from build123d import *

# Parameters (mm, degrees)
F0_W     = 148
F0_H     = 118
F1_DEPTH = 59
F2_R     = 25.75
F3_DEPTH = 50
F2_R_2   = 18
F4_DEPTH = 40
F2_R_3   = 12.5
F5_DEPTH = 38.5
F2_R_4   = 5.4
F6_DEPTH = 38.3


with BuildPart() as f1:
    # F0 (on Top) → F1 (new body)
    with BuildSketch(Plane.XY):
        Rectangle(F0_W, F0_H)
    extrude(amount=F1_DEPTH)

    # F2 (on face) → F3 (cut)
    with BuildSketch(Plane.XY.offset(59)):
        with Locations((0, -26)):
            Circle(F2_R)
    extrude(amount=-F3_DEPTH, mode=Mode.SUBTRACT)

    # F2 (on face) → F4 (cut)
    with BuildSketch(Plane.XY.offset(59)):
        with Locations((-51, 36)):
            Circle(F2_R_2)
        with Locations((0, 36)):
            Circle(F2_R_2)
        with Locations((51, 36)):
            Circle(F2_R_2)
    extrude(amount=-F4_DEPTH, mode=Mode.SUBTRACT)

    # F2 (on face) → F5 (cut)
    with BuildSketch(Plane.XY.offset(59)):
        with Locations((-51, 0)):
            Circle(F2_R_3)
        with Locations((-51, -36)):
            Circle(F2_R_3)
        with Locations((51, 0)):
            Circle(F2_R_3)
        with Locations((51, -36)):
            Circle(F2_R_3)
    extrude(amount=-F5_DEPTH, mode=Mode.SUBTRACT)

    # F2 (on face) → F6 (cut)
    with BuildSketch(Plane.XY.offset(59)):
        with Locations((-24, 13)):
            Circle(F2_R_4)
        with Locations((-36, -18)):
            Circle(F2_R_4)
        with Locations((24, 13)):
            Circle(F2_R_4)
        with Locations((36, -18)):
            Circle(F2_R_4)
    extrude(amount=-F6_DEPTH, mode=Mode.SUBTRACT)


solid = f1.part
Part model, mm, in its own coordinate system. A direction names the side the tool comes from. Coordinates: 2 decimals unless noted, no trailing zeros. Loops run counter-clockwise (first coordinate to the right, second up) from the corner with the lowest first, then second, coordinate; pieces in that order, holes last. Notation, with made-up numbers: M -0.5,6 L 19.5,6 A21 cw 19.5,37 Z; hole C 0.5,36 d7. An arc over 180 degrees is marked long. Use a Markdown table: item, result. Add a question column.
Q1. Cut at B-B (z = 23). Give the number of separate pieces and of enclosed holes in the cut face, and give its area (4 significant figures).
Q2. Pin check, flat tips, straight feed: P1, Ø12.5, axis at x = 49.5, y = -35, coming from the +Z side; P2, Ø5.5, axis at x = 22, y = 13, coming from the +Z side; P3, Ø21.5, axis at x = -51, y = 36, coming from the +Z side. Stop position of each tip, or through.
Q3. Cut at C-C (y = -31.5). Write the cut outline in (x, z), and give its area (3 significant figures).
Q4. Probe L1, parallel to Y at x = 51, z = 40.5; L2, parallel to X at y = -43, z = 30; L3, parallel to X at y = -15, z = 38. List the from-to ranges inside material, lowest first.
Q5. Which spindle directions (+Z, -Z, +X, -X, +Y, -Y) get a long thin tool onto all of the face, cutting with end or side? Do faces 5 (the cylindrical face through (-60.92, -7.606, 40.02)), 6 (the flat face through (-74, -1, 29)). Say none if no direction does.
Q6. Mould opens along Y. For faces 1 (the cylindrical face through (38.512, 0.55, 40.02)), 2 (the flat face through (-1, 59, 29)), 3 (the cylindrical face through (-21.51, 8.21, 40.12)), 4 (the flat face through (74, -1, 29)) say: +Y half, -Y half, draft (parallel to the pull), parting line (faces both ways), or undercut.
Q7. Cut at D-D (x = 0). Write the cut outline in (y, z), and give its area (3 significant figures).
Q8. Cut at A-A (x = 51). Write the cut outline in (y, z).
Worked out:
| question | item | result |
|---|---|---|
| 1 | separate pieces | 1 |
| 1 | enclosed holes | 12 |
| 1 | area | 10,000 mm2 |
| 2 | P1 | stops at z = 20.5 |
| 2 | P2 | stops at z = 20.7 |
| 2 | P3 | stops at z = 19 |
| 3 | outline | M -74,0 L 74,0 L 74,59 L 62.66,59 L 62.66,20.5 L 39.34,20.5 L 39.34,59 L 25.16,59 L 25.16,9 L -25.16,9 L -25.16,59 L -39.34,59 L -39.34,20.5 L -62.66,20.5 L -62.66,59 L -74,59 Z |
| 3 | area | 4,420 mm2 |
| 4 | L1 | y = -59 to -48.5, -23.5 to -12.5, 12.5 to 18, 54 to 59 |
| 4 | L2 | x = -74 to -61.36, -40.64 to -19.34, 19.34 to 40.64, 61.36 to 74 |
| 4 | L3 | x = -74 to -40.49, -31.51 to -23.28, 23.28 to 31.51, 40.49 to 74 |
| 5 | face 5 | +Z |
| 5 | face 6 | +Z, -Z, -X, +Y, -Y |
| 6 | face 1 | undercut |
| 6 | face 2 | +Y half |
| 6 | face 3 | undercut |
| 6 | face 4 | draft |
| 7 | outline | M -59,0 L 59,0 L 59,59 L 54,59 L 54,19 L 18,19 L 18,59 L -0.25,59 L -0.25,9 L -51.75,9 L -51.75,59 L -59,59 Z |
| 7 | area | 2,950 mm2 |
| 8 | outline | M -59,0 L 59,0 L 59,59 L 54,59 L 54,19 L 18,19 L 18,59 L 12.5,59 L 12.5,20.5 L -12.5,20.5 L -12.5,59 L -23.5,59 L -23.5,20.5 L -48.5,20.5 L -48.5,59 L -59,59 Z |
